Design review of the part shown in the three views and the two pictorial views. Dimensions are in mm from the part's minimum x, y and z. A direction names the side the tool comes from. Give positions to 0.01 mm unless a question says otherwise; leave off trailing zeros. Order: outer loops, then holes, each group sorted by start corner. A loop starts at its lowest first (then second) coordinate and runs counter-clockwise, first axis right, second up.
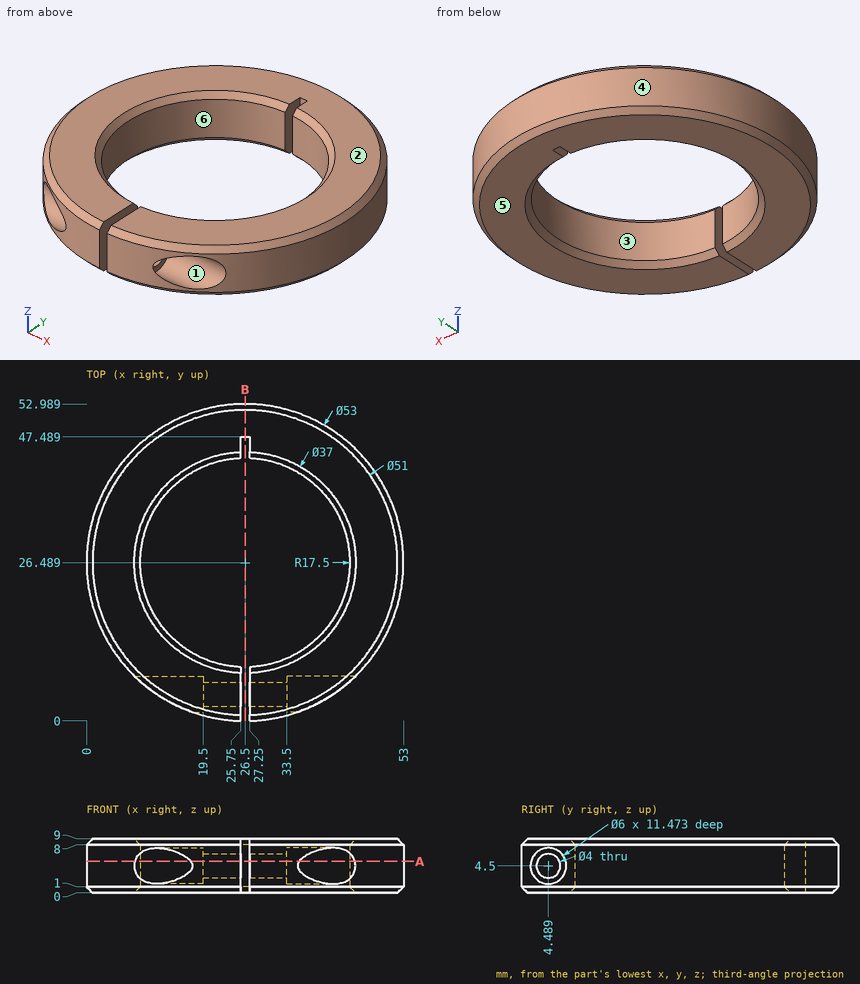
Item 1: Draft analysis for pull direction X (two halves, no side actions). For the marked faces 4, 5 and 6, state which applies: released by +X, released by -X, zero draft, split by the parting line, or undercut.
Values found:
face 4: split by the parting line
face 5: zero draft
face 6: undercut
Item 2: For line 1 (Z direction, x = 31, y = 4.5); line 2 (X direction, y = 26, z = 2.5) (1 decimal); line 3 (Y direction, x = 24.25, z = 4.5) (1 decimal), list the stretches that pass through material, from the lowest coordinate up.
Values found:
line 1: z = 0 to 2.5, 6.5 to 9
line 2: x = 0 to 9, 44 to 53
line 3: y = 0.1 to 2.5, 6.5 to 9.1, 43.8 to 52.9
Item 3: Take a section at B-B (x = 26.5). Give the boundary of the cut face in (y, z), and give its area (3 significant figures).
Values found:
outline: (47.49, 0) - (51.99, 0) - (52.99, 1) - (52.99, 8) - (51.99, 9) - (47.49, 9) - close
area: 48.5 mm2
Item 4: Take a section at A-A (z = 5.25). Give the number of separate pieces and of enclosed holes in the cut face, and give its area (3 significant figures).
Values found:
separate pieces: 3
enclosed holes: 0
area: 1,090 mm2
Item 5: For the marked faces 1, 2 and 3, list the 3-axis set-ups (+Z, -Z, +X, -X, +Y, -Y) from which the entire face can be reached by the end or side of a thin tool; tool diameter is ignored.
Values found:
face 1: +X
face 2: +Z, +X, -X, +Y, -Y
face 3: +Z, -Z
Item 6: Clearance check with flat-ended pins moving along their axes: pin 1 Ø3.5 at (y, z) = (4.49, 4.5) entering from -X; pin 2 Ø4 at (y, z) = (45, 4) entering from +X; pin 3 Ø5 at (y, z) = (16.5, 2.5) entering from +X; pin 4 Ø3 at (y, z) = (46.5, 3.5) entering from -X. State where each tip first meets the part, or that it passes through.
Values found:
pin 1: passes through
pin 2: stops at x = 47.23
pin 3: stops at x = 51.92
pin 4: stops at x = 7.54
